from build123d import *

# Parameters (mm, degrees)
F1_DEPTH     = 5
F2_SIZE2     = 100
F2_SIZE      = 15
F3_W         = 5
F3_H         = 108
F4_DEPTH     = 54
F4_FACE_W    = 5
F4_FACE_H    = 54
F5_ANGLE     = 7.9800839779
F6_W         = 42
F6_H         = 15
F7_DEPTH     = 25
F8_W         = 7.5
F8_H         = 11
F9_DEPTH     = 16
F10_T4_DEPTH = 91.0129088322
F11_R        = 3
F12_W        = 18
F12_H        = 4
F13_DEPTH    = 59
F14_W        = 40
F14_H        = 3
F15_DEPTH    = 38.7
F16_DEPTH    = 15.2
F17_T1_DEPTH = 208.7346390373
F17_T6_DEPTH = 207.8673195186
F18_T4_DEPTH = 299.280483699


# Not quite as in the source:
# - a fillet or chamfer that OpenCascade refuses, or shapes differently, is made with other operations: its cross-section is extruded or revolved along the edge and cut away or added


with BuildPart() as f1:
    # F0 (on Top) → F1 (new body)
    with BuildSketch(Plane.XY):
        with BuildLine():
            Line((57.5, 3.8800953701), (57.5, 61.5))
            Line((57.5, 61.5), (-57.5, 61.5))
            Line((-57.5, 61.5), (-57.5, -61.5))
            Line((-57.5, -61.5), (57.5, -61.5))
            Line((57.5, -61.5), (57.5, -11.1199046299))
            ThreePointArc((57.5, -11.1199046299), (50, -3.6199046299), (57.5, 3.8800953701))
        make_face()
    extrude(amount=F1_DEPTH)

    # F2
    f2_edges = [f1.edges().sort_by_distance(p)[0] for p in [
        (-57.5, 61.5, 2.5),
    ]]
    f2_side = f1.faces().sort_by_distance((-57.5, 0, 2.5))[0]
    chamfer(f2_edges, length=F2_SIZE, length2=F2_SIZE2, reference=f2_side)

    # F3 (on face) → F4 (join)
    with BuildSketch(Plane.XY.offset(5)):
        with Locations((-55, -7.5)):
            Rectangle(F3_W, F3_H)
    extrude(amount=F4_DEPTH)

    # F4_face (on face) → F5 (revolve)
    with BuildSketch(Plane(origin=(-55, 46.5, 32), x_dir=(-1, 0, 0), z_dir=(0, 1, 0))):
        Rectangle(F4_FACE_W, F4_FACE_H)
    revolve(axis=Axis((-57.5, 46.5, 32), (0, 0, 1)), revolution_arc=F5_ANGLE)

    # F6 (on face) → F7 (cut)
    with BuildSketch(Plane.YZ.offset(-52.5)):
        with Locations((-40.5, 51.5)):
            Rectangle(F6_W, F6_H)
    extrude(amount=-F7_DEPTH, mode=Mode.SUBTRACT)

    # F8 (on face) → F9 (join)
    with BuildSketch(Plane(origin=(-57.5, 0, 0), x_dir=(0, -1, 0), z_dir=(-1, 0, 0))):
        with Locations((23.25, 5.5)):
            Rectangle(F8_W, F8_H)
    extrude(amount=F9_DEPTH)

    # F10: chamfer of 16.1 x 6.2 on 1 edges, made by hand


with BuildPart() as f10_tool2:
    # F10_s3 → F10_t4 (new body)
    with BuildSketch(Plane.XZ.offset(68.7564544161)):
        Polygon((-57.4, 11), (-73.5, 4.8), (-73.5, 11), align=None)
    extrude(amount=-F10_T4_DEPTH)

    split(bisect_by=Plane.YZ.offset(-57.5), keep=Keep.BOTTOM)


with BuildPart() as f1_1:
    add(f1.part)

    # F10_t1: cut F10_tool2
    add(f10_tool2.part, mode=Mode.SUBTRACT)

    # F11
    f11_edges = [f1_1.edges().sort_by_distance(p)[0] for p in [
        (-65.5, -27, 7.880745),
        (-65.5, -19.5, 7.880745),
    ]]
    fillet(f11_edges, radius=F11_R)

    # F12 (on Top) → F13 (join)
    with BuildSketch(Plane.XY):
        with Locations((-61.6593700051, 45.0587611198)):
            Rectangle(F12_W, F12_H)
    extrude(amount=F13_DEPTH)

    # F14 (on face) → F15 (join)
    with BuildSketch(Plane.XY.offset(5)):
        with Locations((-32.5, -60)):
            Rectangle(F14_W, F14_H)
        with Locations((-32.5, 45)):
            Rectangle(F14_W, F14_H)
    extrude(amount=F15_DEPTH)

    # F16 (add): a face of the model
    f16_faces = [f1_1.faces().sort_by_distance(p)[0] for p in [
        (-32.5, 45, 43.7),
    ]]
    extrude(f16_faces, amount=F16_DEPTH)

    # F17: chamfer of 40 on 2 edges, made by hand

    # F17_s2 → F17_t1 (cut)
    with BuildSketch(Plane.XZ.offset(-149.3673195186)):
        Polygon((-52.5, 58.9), (-12.5, 18.9), (-12.5, 58.9), align=None)
    extrude(amount=F17_T1_DEPTH, mode=Mode.SUBTRACT)


with BuildPart() as f17_tool4:
    # F17_s5 → F17_t6 (new body)
    with BuildSketch(Plane.XZ.offset(164.3673195186)):
        Polygon((-52.5, 43.7), (-12.5, 3.7), (-12.5, 43.7), align=None)
    extrude(amount=-F17_T6_DEPTH)

    split(bisect_by=Plane.XY.offset(5), keep=Keep.TOP)


with BuildPart() as f1_2:
    add(f1_1.part)

    # F17_t3: cut F17_tool4
    add(f17_tool4.part, mode=Mode.SUBTRACT)

    # F18: chamfer of 14.1 x 57 on 1 edges, made by hand


with BuildPart() as f18_tool2:
    # F18_s3 → F18_t4 (new body)
    with BuildSketch(Plane.XZ.offset(-194.6402418495)):
        Polygon((-52.8050865276, 59.2050865276), (-12.5, 4.8), (-12.5, 18.9), align=None)
    extrude(amount=F18_T4_DEPTH)

    split(bisect_by=Plane.XY.offset(5), keep=Keep.TOP)

    split(bisect_by=Plane.YZ.offset(-52.5), keep=Keep.TOP)


with BuildPart() as f1_3:
    add(f1_2.part)

    # F18_t1: cut F18_tool2
    add(f18_tool2.part, mode=Mode.SUBTRACT)


solid = f1_3.part
Work out the finished part from the listing and answer in its coordinate system (mm). A direction names the side the tool comes from. Round coordinates to 2 decimals unless told otherwise and drop trailing zeros. Order: outer loops, then holes, each group sorted by start corner. A loop starts at its lowest first (then second) coordinate and runs counter-clockwise, first axis right, second up. Notation, with made-up numbers: M -10.75,-10.75 L 34.25,-10.75 A27 ccw 34.25,28.25 Z; hole C 82,-23 d9. An arc over 180 degrees is marked long. Put each result on its own line as item: value. Start each with the question number.
Q1. Straight lines are drawn through the part: L1, parallel to Y at x = -39, z = 6.5; L2, parallel to X at y = 28, z = 13.5; L3, parallel to Z at x = 7.5, y = 13. For each, find the intervals that lie inside material, in ascending order. Write a range as [from, to].
Q2. Flat-ended cylindrical pins translate along their axes: pin 1 (10 mm diameter, centred on x = -23, y = -6.5, fed in from -Z); pin 2 (8 mm diameter, centred on x = -59, z = 47, fed in from +Y); pin 3 (5 mm diameter, centred on y = -31, z = 33.5, fed in from +X); pin 4 (1.2 mm diameter, centred on y = 46, z = 27.5, fed in from -X). Find the tip coordinate at first contact, or state that the pin passes through.
Q3. Section B-B, the plane z = 24 is taken. Write down the section's boundary in (x, y).
Q4. Section D-D, the plane z = 33 is taken. Write down the section's boundary in (x, y).
Q5. Section C-C, the plane x = -31 is taken. Write down the section's boundary in (y, z) (3 decimals).
Q6. Section A-A, the plane y = 9.5 is taken. Write down the section's boundary in (x, z).
Q7. A tool of negligible diameter and unlimited length cuts with its end or side. For faces 4 (the flat face through (-33.4, -60, 24.6)), 5 (the flat face through (-55, -19.5, 51)), 6 (the flat face through (-64, -19.5, 3)), 7 (the flat face through (-52.5, -8, 32)), from which of +Z, -Z, +X, -X, +Y, -Y can it reach the whole face along a straight path? Write none if from no direction.
Q8. For a pull along Y with two mould halves and no side action, classify faces 1 (the flat face through (-37, 46.5, 26)), 2 (the flat face through (-65.388, -23.26, 7.924)), 3 (the cylindrical face through (-65.61, -20.4, 6.92)) as pulls with the +Y half, pulls with the -Y half, needs draft (parallel to the pull), parting line crosses it, or undercut.
Findings below:
1. L1: y = [-61.5, -58.5], [43.5, 46.5]
1. L2: x = [-57.5, -52.5]
1. L3: z = [0, 5]
2. pin 1: stops at z = 0
2. pin 2: stops at y = 47.06
2. pin 3: stops at x = -52.5
2. pin 4: stops at x = -70.66
3. outline: M -70.66,43.06 L -57.5,43.06 L -57.5,-61.5 L -32.8,-61.5 L -32.8,-58.5 L -52.5,-58.5 L -52.5,43.5 L -26.72,43.5 L -26.72,46.5 L -52.5,46.5 A5 ccw -52.55,47.19 L -53.51,47.06 L -70.66,47.06 Z
4. outline: M -70.66,43.06 L -57.5,43.06 L -57.5,-61.5 L -41.8,-61.5 L -41.8,-58.5 L -52.5,-58.5 L -52.5,43.5 L -33.39,43.5 L -33.39,46.5 L -52.5,46.5 A5 ccw -52.55,47.19 L -53.51,47.06 L -70.66,47.06 Z
5. outline: M -61.5,0 L 50.475,0 L 50.475,5 L 46.5,5 L 46.5,29.772 L 43.5,29.772 L 43.5,5 L -58.5,5 L -58.5,22.2 L -61.5,22.2 Z
6. outline: M -57.5,0 L 57.5,0 L 57.5,5 L -52.5,5 L -52.5,59 L -57.5,59 Z
7. face 4: +Z, +X, -Y
7. face 5: +Z, +X, -X, -Y
7. face 6: +Z, -Z, -X
7. face 7: +Z, +X
8. face 1: pulls with the +Y half
8. face 2: needs draft
8. face 3: undercut
